Design review of the part built by this model. Coordinates are the model's own, in mm. A direction names the side the tool comes from. Give positions to 0.01 mm unless a question says otherwise; leave off trailing zeros. Write each loop counter-clockwise with the first axis right and the second up, starting at its lowest first coordinate (ties: lowest second). Pieces come first, ordered by that corner, then holes. Notation, with made-up numbers: M 8,-40 L 20,-40 A28 cw 20,-21 Z; hole C 87,-15 d6. An arc over 180 degrees is marked long. Answer in a Markdown table with one row per item.
```python
from build123d import *

# Parameters (mm, degrees)
SKETCH_1_W          = 28
SKETCH_1_H          = 12
EXTRUDE_1_DEPTH     = 21
SKETCH_2_R          = 1.75
CUT_EXTRUDE_1_DEPTH = 59
SKETCH_3_R          = 2.2
CUT_EXTRUDE_2_DEPTH = 65
SKETCH_7_W          = 15
SKETCH_7_H          = 15
CUT_EXTRUDE_3_DEPTH = 109
CUT_EXTRUDE_5_DEPTH = 84
FILLET_1_R          = 2
CUT_EXTRUDE_6_DEPTH = 6
SKETCH_15_W         = 25
SKETCH_15_H         = 16
CUT_EXTRUDE_7_DEPTH = 55
FILLET_2_R          = 4


with BuildPart() as part:
    # 草图1 → 凸台-拉伸1 (new body)
    with BuildSketch(Plane.XY):
        Polygon((56, -12), (28, -12), (0, -12), (-13, -12), (-13, -63), (69, -63), (69, -12), align=None)
        with Locations((42, -6)):
            Rectangle(SKETCH_1_W, SKETCH_1_H)
        with Locations((14, -6)):
            Rectangle(SKETCH_1_W, SKETCH_1_H)
    extrude(amount=EXTRUDE_1_DEPTH)

    # 草图2 → 切除-拉伸1 (cut)
    with BuildSketch(Plane(origin=(0, 0, 0), x_dir=(-1, 0, 0), z_dir=(0, 0, -1))):
        with Locations((-58, -54.25)):
            Circle(SKETCH_2_R)
        with Locations((2, -54.25)):
            Circle(SKETCH_2_R)
    extrude(amount=-CUT_EXTRUDE_1_DEPTH, mode=Mode.SUBTRACT)

    # 草图3 → 切除-拉伸2 (cut)
    with BuildSketch(Plane(origin=(0, 0, 0), x_dir=(1, 0, 0), z_dir=(0, 1, 0))):
        with Locations(Location((48.5, -10.5, 0), (0, 0, 180))):
            Circle(SKETCH_3_R)
        with Locations(Location((8.5, -10.5, 0), (0, 0, 180))):
            Circle(SKETCH_3_R)
    extrude(amount=-CUT_EXTRUDE_2_DEPTH, mode=Mode.SUBTRACT)

    # 草图7 → 切除-拉伸3 (cut)
    with BuildSketch(Plane(origin=(69, 0, 0), x_dir=(0, 0, -1), z_dir=(1, 0, 0))):
        with Locations((-10.5, -19.5)):
            Rectangle(SKETCH_7_W, SKETCH_7_H)
    extrude(amount=-CUT_EXTRUDE_3_DEPTH, mode=Mode.SUBTRACT)

    # 草图9 → 切除-拉伸5 (cut, symmetric)
    with BuildSketch(Plane(origin=(56, 0, 0), x_dir=(0, 0, -1), z_dir=(1, 0, 0))):
        Polygon((-18, -27), (-18, -12), (-21, -12), (-21, -63), (0, -63), (0, -12), (-3, -12), (-3, -27), align=None)
    extrude(amount=CUT_EXTRUDE_5_DEPTH, both=True, mode=Mode.SUBTRACT)

    # 圆角1
    fillet_1_edges = [part.edges().sort_by_distance(p)[0] for p in [
        (0, -6, 0),
        (56, -6, 0),
        (56, -6, 21),
        (0, -6, 21),
    ]]
    fillet(fillet_1_edges, radius=FILLET_1_R)

    # 草图14 → 切除-拉伸6 (cut)
    with BuildSketch(Plane(origin=(0, 0, 0), x_dir=(1, 0, 0), z_dir=(0, 1, 0))):
        with BuildLine():
            Line((56, -19), (56, -2))
            ThreePointArc((56, -2), (55.414213562, -0.585786438), (54, 0))
            Line((54, 0), (2, 0))
            ThreePointArc((2, 0), (0.585786438, -0.585786438), (0, -2))
            Line((0, -2), (0, -19))
            ThreePointArc((0, -19), (0.585786438, -20.414213562), (2, -21))
            Line((2, -21), (54, -21))
            ThreePointArc((54, -21), (55.414213562, -20.414213562), (56, -19))
        make_face()
    extrude(amount=-CUT_EXTRUDE_6_DEPTH, mode=Mode.SUBTRACT)

    # 草图15 → 切除-拉伸7 (cut)
    with BuildSketch(Plane(origin=(0, -6, 0), x_dir=(1, 0, 0), z_dir=(0, 1, 0))):
        with Locations((28, -10.5)):
            Rectangle(SKETCH_15_W, SKETCH_15_H)
    extrude(amount=-CUT_EXTRUDE_7_DEPTH, mode=Mode.SUBTRACT)

    # 圆角2
    fillet_2_edges = [part.edges().sort_by_distance(p)[0] for p in [
        (40.5, -9, 2.5),
        (40.5, -9, 18.5),
        (15.5, -9, 18.5),
        (15.5, -9, 2.5),
    ]]
    fillet(fillet_2_edges, radius=FILLET_2_R)


solid = part.part
```
1) Add section C-C (z = 10.5). Write out the cut boundary in (x, y).
Geometry says:
| item | result |
|---|---|
| outline | M 0,-12 L 6.3,-12 L 6.3,-6 L 0,-6 Z; M 10.7,-12 L 15.5,-12 L 15.5,-6 L 10.7,-6 Z; M 40.5,-12 L 46.3,-12 L 46.3,-6 L 40.5,-6 Z; M 50.7,-12 L 56,-12 L 56,-6 L 50.7,-6 Z |
2) To check wall thickness, follow probe 1 along X at (y, z) = (-8.25, 7.5); probe 2 along Z at (x, y) = (48.5, -9.85); probe 3 along Z at (x, y) = (22, -11.1). State the ranges of each line that lie inside material, in increasing order. Write a range as [from, to].
Geometry says:
| item | result |
|---|---|
| probe 1 | [0, 15.5], [40.5, 56] |
| probe 2 | [0, 8.3], [12.7, 21] |
| probe 3 | [0, 2.5], [18.5, 21] |
3) Add section D-D (z = 16.25). Write out the cut boundary in (x, y), and give its area (3 significant figures).
Geometry says:
| item | result |
|---|---|
| outline | M 0,-12 L 15.9,-12 L 15.9,-6 L 0,-6 Z; M 40.1,-12 L 56,-12 L 56,-6 L 40.1,-6 Z |
| area | 191 mm^2 |
4) For faces 1 (the face through (28, -9, 2.5)), 2 (the face through (28, -6, 1)), list the 3-axis set-ups (+Z, -Z, +X, -X, +Y, -Y) from which the entire face can be reached by the end or side of a thin tool; tool diameter is ignored.
Geometry says:
| item | result |
|---|---|
| face 1 | +Y, -Y |
| face 2 | +Z, -Z, +X, -X, +Y |
5) The part is to be moulded in two halves that separate along Z. For faces 3 (the face through (56, -9, 10)), 4 (the face through (39.297, -9.042, 17.359)), 5 (the face through (28, -9, 0)), say which applies: released by +Z, released by -Z, zero draft, split by the parting line, or undercut.
Geometry says:
| item | result |
|---|---|
| face 3 | zero draft |
| face 4 | undercut |
| face 5 | released by -Z |
6) Add section B-B (y = -9.85). Write out the cut boundary in (x, z).
Geometry says:
| item | result |
|---|---|
| outline | M 0,2 A2 ccw 2,0 L 54,0 A2 ccw 56,2 L 56,19 A2 ccw 54,21 L 2,21 A2 ccw 0,19 Z; hole C 8.5,10.5 d4.4; hole M 15.5,6.5 A4 ccw 19.5,2.5 L 36.5,2.5 A4 ccw 40.5,6.5 L 40.5,14.5 A4 ccw 36.5,18.5 L 19.5,18.5 A4 ccw 15.5,14.5 Z; hole C 48.5,10.5 d4.4 |
7) Add section A-A (x = 24.5). Write out the cut boundary in (y, z), and give its area (3 significant figures).
Geometry says:
| item | result |
|---|---|
| outline | M -12,0 L -6,0 L -6,2.5 L -12,2.5 Z; M -12,18.5 L -6,18.5 L -6,21 L -12,21 Z |
| area | 30.0 mm^2 |
